from build123d import *

# Parameters (mm, degrees)
BOSS_EXTRUDE1_DEPTH     = 42
CUT_EXTRUDE1_DEPTH      = 54.409262615
CUT_EXTRUDE1_DEPTH_BACK = 54.409262615
SKETCH4_R               = 1.6
SKETCH5_R               = 3.1
CUT_EXTRUDE2_DEPTH      = 69.909723571


with BuildPart() as part:
    # Sketch1 → Boss-Extrude1 (new body)
    with BuildSketch(Plane.XY):
        Polygon((-26.186542305, -22.524647199), (-7.843396555, -22.524647199), (-7.843396555, -26.524647199), (-27.843396555, -26.524647199), (-49.05659999, -5.311443763), (-46.228172865, -2.483016639), align=None)
    extrude(amount=BOSS_EXTRUDE1_DEPTH)

    # Sketch4 → Cut-Extrude1 (cut, two sides: drawn at the far end of the back side and taken through both)
    with BuildSketch(Plane(origin=(-27.184021877, -27.184021877, 0), x_dir=(0, 0, 1), z_dir=(-0.7071067811865462, -0.707106781186549, 0)).offset(-CUT_EXTRUDE1_DEPTH_BACK)):
        with Locations(Location((31, 23.932496612, 0), (0, 0, 270))):
            Circle(SKETCH4_R)
        with Locations(Location((11, 23.932496612, 0), (0, 0, 270))):
            Circle(SKETCH4_R)
    extrude(amount=CUT_EXTRUDE1_DEPTH + CUT_EXTRUDE1_DEPTH_BACK, mode=Mode.SUBTRACT)

    # Sketch5 → Cut-Extrude2 (cut, through all)
    with BuildSketch(Plane.XZ.offset(26.524647199)):
        with Locations((-17.843396555, 33)):
            Circle(SKETCH5_R)
        with Locations((-17.843396555, 9)):
            Circle(SKETCH5_R)
    extrude(amount=-CUT_EXTRUDE2_DEPTH, mode=Mode.SUBTRACT)


solid = part.part
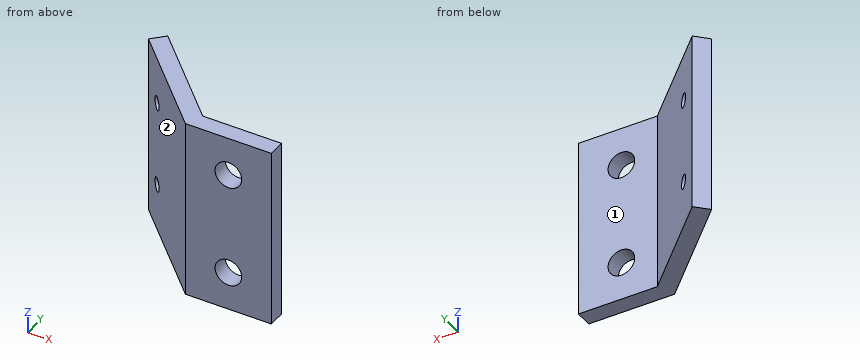
Geometry check sheet. Reference: the model listing, model coordinates, mm. Face numbers are marked on the shaded views. A direction names the side the tool comes from. Round coordinates to 2 decimals unless told otherwise and drop trailing zeros. Write each loop counter-clockwise with the first axis right and the second up, starting at its lowest first coordinate (ties: lowest second). Pieces come first, ordered by that corner, then holes.
Item 1: Access from +Z, -Z, +X, -X, +Y, -Y to the whole of each face (thin tool, end or side, straight path). Record for the marked faces 1 and 2.
Determined:
face 1: +Z, -Z, +X, +Y
face 2: +Z, -Z, -X, -Y
Item 2: Go/stop test with flat-tipped pins: pin 1 Ø12 at (y, z) = (-21, 16.5) entering from -X; pin 2 Ø14.5 at (x, z) = (-19.5, 16.5) entering from +Y; pin 3 Ø5 at (y, z) = (-18, 11) entering from -X. Record where each tip stops, or that it passes through.
Determined:
pin 1: stops at x = -39.37
pin 2: stops at y = -21.96
pin 3: stops at x = -38.87
Item 3: Section check B-B (x = -22). Record the boundary of the cut face in (y, z), plus the area to 3 significant figures.
Determined:
outline: (-26.52, 0) - (-22.52, 0) - (-22.52, 42) - (-26.52, 42) - close
area: 168 mm2
Item 4: Section check C-C (y = -20.5). Record the boundary of the cut face in (x, z).
Determined:
outline: (-33.87, 0) - (-28.21, 0) - (-28.21, 42) - (-33.87, 42) - close
Item 5: Section check A-A (z = 4). Record the boundary of the cut face in (x, y).
Determined:
outline: (-49.06, -5.31) - (-27.84, -26.52) - (-7.84, -26.52) - (-7.84, -22.52) - (-26.19, -22.52) - (-46.23, -2.48) - close
Item 6: Material ranges on line 1 along Y through (x, z) = (-19.5, 36.5); line 2 along X through (y, z) = (-11.5, 18); line 3 along Y through (x, z) = (-42.5, 25), recorded low to high.
Determined:
line 1: y = -26.52 to -22.52
line 2: x = -42.87 to -37.21
line 3: y = -11.87 to -6.21
